Autodesk Inventor part; units mm, degrees
ref_plane "YZ Plane" through (0, 0, 0) normal (1, 0, 0) x (0, 1, 0)
ref_plane "XZ Plane" through (0, 0, 0) normal (0, 1, 0) x (-1, 0, 0)
ref_plane "XY Plane" through (0, 0, 0) normal (0, 0, 1) x (1, 0, 0)
sketch "Block1" plane through (0, 0, 0) normal (0, 0, 1) x (1, 0, 0)
  line L0 (-23.62, 29.22) -> (-7.58, 29.22)
  line L1 (-7.58, 29.22) -> (-7.58, 20.22)
  line L2 (-7.58, 20.22) -> (7.58, 20.22)
  line L3 (7.58, 20.22) -> (7.58, 29.22)
  line L4 (7.58, 29.22) -> (23.62, 29.22)
  line L5 (23.62, 29.22) -> (23.62, 20.22)
  line L6 (23.62, 20.22) -> (39.22, 20.22)
  line L7 (39.22, 20.22) -> (39.22, 13.1133)
  line L8 (39.22, 13.1133) -> (30.22, 13.1133)
  line L9 (30.22, 13.1133) -> (30.22, 5.5533)
  line L10 (30.22, 5.5533) -> (39.22, 5.5533)
  line L11 (39.22, 5.5533) -> (39.22, -5.5533)
  line L12 (39.22, -5.5533) -> (30.22, -5.5533)
  line L13 (30.22, -5.5533) -> (30.22, -13.1133)
  line L14 (30.22, -13.1133) -> (39.22, -13.1133)
  line L15 (39.22, -13.1133) -> (39.22, -20.22)
  line L16 (39.22, -20.22) -> (-39.22, -20.22)
  line L17 (-39.22, -20.22) -> (-39.22, -13.1133)
  line L18 (-39.22, -13.1133) -> (-30.22, -13.1133)
  line L19 (-30.22, -13.1133) -> (-30.22, -5.5533)
  line L20 (-30.22, -5.5533) -> (-39.22, -5.5533)
  line L21 (-39.22, -5.5533) -> (-39.22, 5.5533)
  line L22 (-39.22, 5.5533) -> (-30.22, 5.5533)
  line L23 (-30.22, 5.5533) -> (-30.22, 13.1133)
  line L24 (-30.22, 13.1133) -> (-39.22, 13.1133)
  line L25 (-39.22, 13.1133) -> (-39.22, 20.22)
  line L26 (-39.22, 20.22) -> (-23.62, 20.22)
  line L27 (-23.62, 20.22) -> (-23.62, 29.22)
  line L28 (4.22, 8.55) -> (4.22, 3.11)
  line L29 (4.22, 3.11) -> (-4.22, 3.11)
  line L30 (-4.22, 3.11) -> (-4.22, 8.55)
  line L31 (-4.22, 8.55) -> (4.22, 8.55)
  line L32 (4.22, -3.11) -> (4.22, -8.55)
  line L33 (4.22, -8.55) -> (-4.22, -8.55)
  line L34 (-4.22, -8.55) -> (-4.22, -3.11)
  line L35 (-4.22, -3.11) -> (4.22, -3.11)
  point P0 (0, 5.4933)
sketch "Block2" plane through (0, 0, 0) normal (0, 0, 1) x (1, 0, 0)
  line L0 (-23.5, 29.1) -> (-7.7, 29.1)
  line L1 (-7.7, 29.1) -> (-7.7, 20.1)
  line L2 (-7.7, 20.1) -> (7.7, 20.1)
  line L3 (7.7, 20.1) -> (7.7, 29.1)
  line L4 (7.7, 29.1) -> (23.5, 29.1)
  line L5 (23.5, 29.1) -> (23.5, 20.1)
  line L6 (23.5, 20.1) -> (39.1, 20.1)
  line L7 (39.1, 20.1) -> (39.1, 13.2333)
  line L8 (39.1, 13.2333) -> (30.1, 13.2333)
  line L9 (30.1, 13.2333) -> (30.1, 5.4333)
  line L10 (30.1, 5.4333) -> (39.1, 5.4333)
  line L11 (39.1, 5.4333) -> (39.1, -5.4333)
  line L12 (39.1, -5.4333) -> (30.1, -5.4333)
  line L13 (30.1, -5.4333) -> (30.1, -13.2333)
  line L14 (30.1, -13.2333) -> (39.1, -13.2333)
  line L15 (39.1, -13.2333) -> (39.1, -20.1)
  line L16 (39.1, -20.1) -> (-39.1, -20.1)
  line L17 (-39.1, -20.1) -> (-39.1, -13.2333)
  line L18 (-39.1, -13.2333) -> (-30.1, -13.2333)
  line L19 (-30.1, -13.2333) -> (-30.1, -5.4333)
  line L20 (-30.1, -5.4333) -> (-39.1, -5.4333)
  line L21 (-39.1, -5.4333) -> (-39.1, 5.4333)
  line L22 (-39.1, 5.4333) -> (-30.1, 5.4333)
  line L23 (-30.1, 5.4333) -> (-30.1, 13.2333)
  line L24 (-30.1, 13.2333) -> (-39.1, 13.2333)
  line L25 (-39.1, 13.2333) -> (-39.1, 20.1)
  line L26 (-39.1, 20.1) -> (-23.5, 20.1)
  line L27 (-23.5, 20.1) -> (-23.5, 29.1)
  line L28 (4.1, 8.43) -> (4.1, 3.23)
  line L29 (4.1, 3.23) -> (-4.1, 3.23)
  line L30 (-4.1, 3.23) -> (-4.1, 8.43)
  line L31 (-4.1, 8.43) -> (4.1, 8.43)
  line L32 (4.1, -3.23) -> (4.1, -8.43)
  line L33 (4.1, -8.43) -> (-4.1, -8.43)
  line L34 (-4.1, -8.43) -> (-4.1, -3.23)
  line L35 (-4.1, -3.23) -> (4.1, -3.23)
  point P0 (0, 5.4667)
sketch "Block3" plane through (0, 0, 0) normal (0, 0, 1) x (1, 0, 0)
  line L0 (7.6, 29.2) -> (23.6, 29.2)
  line L1 (23.6, 29.2) -> (23.6, 20.2)
  line L2 (23.6, 20.2) -> (39.2, 20.2)
  line L3 (39.2, 20.2) -> (39.2, 13.1333)
  line L4 (39.2, 13.1333) -> (30.2, 13.1333)
  line L5 (30.2, 13.1333) -> (30.2, 5.5333)
  line L6 (30.2, 5.5333) -> (39.2, 5.5333)
  line L7 (39.2, 5.5333) -> (39.2, -5.5333)
  line L8 (39.2, -5.5333) -> (30.2, -5.5333)
  line L9 (30.2, -5.5333) -> (30.2, -13.1333)
  line L10 (30.2, -13.1333) -> (39.2, -13.1333)
  line L11 (39.2, -13.1333) -> (39.2, -20.2)
  line L12 (39.2, -20.2) -> (-39.2, -20.2)
  line L13 (-39.2, -20.2) -> (-39.2, -13.1333)
  line L14 (-39.2, -13.1333) -> (-30.2, -13.1333)
  line L15 (-30.2, -13.1333) -> (-30.2, -5.5333)
  line L16 (-30.2, -5.5333) -> (-39.2, -5.5333)
  line L17 (-39.2, -5.5333) -> (-39.2, 5.5333)
  line L18 (-39.2, 5.5333) -> (-30.2, 5.5333)
  line L19 (-30.2, 5.5333) -> (-30.2, 13.1333)
  line L20 (-30.2, 13.1333) -> (-39.2, 13.1333)
  line L21 (-39.2, 13.1333) -> (-39.2, 20.2)
  line L22 (-39.2, 20.2) -> (-23.6, 20.2)
  line L23 (-23.6, 20.2) -> (-23.6, 29.2)
  line L24 (-23.6, 29.2) -> (-7.6, 29.2)
  line L25 (-7.6, 29.2) -> (-7.6, 20.2)
  line L26 (-7.6, 20.2) -> (7.6, 20.2)
  line L27 (7.6, 20.2) -> (7.6, 29.2)
  line L28 (4.2, 8.53) -> (4.2, 3.13)
  line L29 (4.2, 3.13) -> (-4.2, 3.13)
  line L30 (-4.2, 3.13) -> (-4.2, 8.53)
  line L31 (-4.2, 8.53) -> (4.2, 8.53)
  line L32 (4.2, -3.13) -> (4.2, -8.53)
  line L33 (4.2, -8.53) -> (-4.2, -8.53)
  line L34 (-4.2, -8.53) -> (-4.2, -3.13)
  line L35 (-4.2, -3.13) -> (4.2, -3.13)
  point P0 (0, 5.4889)
sketch "Block4" plane through (0, 0, 0) normal (0, 0, 1) x (1, 0, 0)
  line L0 (7.7, 29.1) -> (23.5, 29.1)
  line L1 (23.5, 29.1) -> (23.5, 20.1)
  line L2 (23.5, 20.1) -> (39.1, 20.1)
  line L3 (39.1, 20.1) -> (39.1, 13.2333)
  line L4 (39.1, 13.2333) -> (30.1, 13.2333)
  line L5 (30.1, 13.2333) -> (30.1, 5.4333)
  line L6 (30.1, 5.4333) -> (39.1, 5.4333)
  line L7 (39.1, 5.4333) -> (39.1, -5.4333)
  line L8 (39.1, -5.4333) -> (30.1, -5.4333)
  line L9 (30.1, -5.4333) -> (30.1, -13.2333)
  line L10 (30.1, -13.2333) -> (39.1, -13.2333)
  line L11 (39.1, -13.2333) -> (39.1, -20.1)
  line L12 (39.1, -20.1) -> (-39.1, -20.1)
  line L13 (-39.1, -20.1) -> (-39.1, -13.2333)
  line L14 (-39.1, -13.2333) -> (-30.1, -13.2333)
  line L15 (-30.1, -13.2333) -> (-30.1, -5.4333)
  line L16 (-30.1, -5.4333) -> (-39.1, -5.4333)
  line L17 (-39.1, -5.4333) -> (-39.1, 5.4333)
  line L18 (-39.1, 5.4333) -> (-30.1, 5.4333)
  line L19 (-30.1, 5.4333) -> (-30.1, 13.2333)
  line L20 (-30.1, 13.2333) -> (-39.1, 13.2333)
  line L21 (-39.1, 13.2333) -> (-39.1, 20.1)
  line L22 (-39.1, 20.1) -> (-23.5, 20.1)
  line L23 (-23.5, 20.1) -> (-23.5, 29.1)
  line L24 (-23.5, 29.1) -> (-7.7, 29.1)
  line L25 (-7.7, 29.1) -> (-7.7, 20.1)
  line L26 (-7.7, 20.1) -> (7.7, 20.1)
  line L27 (7.7, 20.1) -> (7.7, 29.1)
  line L28 (4.1, 8.43) -> (4.1, 3.23)
  line L29 (4.1, 3.23) -> (-4.1, 3.23)
  line L30 (-4.1, 3.23) -> (-4.1, 8.43)
  line L31 (-4.1, 8.43) -> (4.1, 8.43)
  line L32 (4.1, -3.23) -> (4.1, -8.43)
  line L33 (4.1, -8.43) -> (-4.1, -8.43)
  line L34 (-4.1, -8.43) -> (-4.1, -3.23)
  line L35 (-4.1, -3.23) -> (4.1, -3.23)
  point P0 (0, 5.4667)
sketch "Block5" plane through (0, 0, 0) normal (0, 0, 1) x (1, 0, 0)
  line L0 (-21.38, 25.58) -> (-7.02, 25.58)
  line L1 (-7.02, 25.58) -> (-7.02, 20.08)
  line L2 (-7.02, 20.08) -> (7.02, 20.08)
  line L3 (7.02, 20.08) -> (7.02, 25.58)
  line L4 (7.02, 25.58) -> (21.38, 25.58)
  line L5 (21.38, 25.58) -> (21.38, 20.08)
  line L6 (21.38, 20.08) -> (35.58, 20.08)
  line L7 (35.58, 20.08) -> (35.58, 13.2533)
  line L8 (35.58, 13.2533) -> (30.08, 13.2533)
  line L9 (30.08, 13.2533) -> (30.08, 5.4133)
  line L10 (30.08, 5.4133) -> (35.58, 5.4133)
  line L11 (35.58, 5.4133) -> (35.58, -5.4133)
  line L12 (35.58, -5.4133) -> (30.08, -5.4133)
  line L13 (30.08, -5.4133) -> (30.08, -13.2533)
  line L14 (30.08, -13.2533) -> (35.58, -13.2533)
  line L15 (35.58, -13.2533) -> (35.58, -20.08)
  line L16 (35.58, -20.08) -> (-35.58, -20.08)
  line L17 (-35.58, -20.08) -> (-35.58, -13.2533)
  line L18 (-35.58, -13.2533) -> (-30.08, -13.2533)
  line L19 (-30.08, -13.2533) -> (-30.08, -5.4133)
  line L20 (-30.08, -5.4133) -> (-35.58, -5.4133)
  line L21 (-35.58, -5.4133) -> (-35.58, 5.4133)
  line L22 (-35.58, 5.4133) -> (-30.08, 5.4133)
  line L23 (-30.08, 5.4133) -> (-30.08, 13.2533)
  line L24 (-30.08, 13.2533) -> (-35.58, 13.2533)
  line L25 (-35.58, 13.2533) -> (-35.58, 20.08)
  line L26 (-35.58, 20.08) -> (-21.38, 20.08)
  line L27 (-21.38, 20.08) -> (-21.38, 25.58)
  line L28 (4.08, 8.41) -> (4.08, 3.25)
  line L29 (4.08, 3.25) -> (-4.08, 3.25)
  line L30 (-4.08, 3.25) -> (-4.08, 8.41)
  line L31 (-4.08, 8.41) -> (4.08, 8.41)
  line L32 (4.08, -3.25) -> (4.08, -8.41)
  line L33 (4.08, -8.41) -> (-4.08, -8.41)
  line L34 (-4.08, -8.41) -> (-4.08, -3.25)
  line L35 (-4.08, -3.25) -> (4.08, -3.25)
  point P0 (0, 5.0733)
sketch "Sketch1" plane through (0, 0, 0) normal (0, 0, 1) x (1, 0, 0)
  line L0 (35.5, -20) -> (-35.5, -20)
  line L1 (-35.5, -20) -> (-35.5, 20)
  line L2 (-35.5, 20) -> (35.5, 20)
  line L3 (35.5, 20) -> (35.5, -20)
  line L4 (35.5, -20) -> (-35.5, 20) construction
  line L5 (-35.5, -20) -> (35.5, 20) construction
  point P0 (0, 0)
  point P1 (0, 0)
  dimension "d0" = 71
  dimension "d1" = 40
extrude "Extrusion1" add sketch "Sketch1" against normal blind 5.5
sketch "Sketch3" plane through (0, 0, 0) normal (0, 0, 1) x (1, 0, 0)
  line L0 (-35.5, 20) -> (35.5, 20)
  line L1 (-35.5, -20) -> (-35.5, 20)
  line L2 (-35.5, 13.3333) -> (-30, 13.3333)
  line L3 (-30, 13.3333) -> (-30, 5.3333)
  line L4 (-30, 5.3333) -> (-35.5, 5.3333)
  line L5 (-35.5, 13.3333) -> (-35.5, 5.3333)
  line L6 (-161.1974, 0) -> (72.4829, 0)
  line L7 (0, -29.94) -> (0, 38.94)
  line L8 (35.5, 13.3333) -> (30, 13.3333)
  line L9 (30, 13.3333) -> (30, 5.3333)
  line L10 (30, 5.3333) -> (35.5, 5.3333)
  line L11 (35.5, 13.3333) -> (35.5, 5.3333)
  line L12 (-35.5, -13.3333) -> (-30, -13.3333)
  line L13 (-30, -13.3333) -> (-30, -5.3333)
  line L14 (-30, -5.3333) -> (-35.5, -5.3333)
  line L15 (-35.5, -13.3333) -> (-35.5, -5.3333)
  line L16 (30, -13.3333) -> (30, -5.3333)
  line L17 (35.5, -13.3333) -> (35.5, -5.3333)
  line L18 (30, -5.3333) -> (35.5, -5.3333)
  line L19 (35.5, -13.3333) -> (30, -13.3333)
  point P0 (0, 0)
  dimension "d16" = 5.5
  dimension "d17" = 8
  dimension "d18" = 6.6667
sketch "Sketch4" plane through (0, 0, 0) normal (0, 0, 1) x (1, 0, 0)
  line L0 (4, -8.33) -> (-4, -8.33)
  line L1 (-4, -8.33) -> (-4, -3.33)
  line L2 (-4, -3.33) -> (4, -3.33)
  line L3 (4, -3.33) -> (4, -8.33)
  line L4 (4, -8.33) -> (-4, -3.33) construction
  line L5 (-4, -8.33) -> (4, -3.33) construction
  line L6 (-161.1974, 0) -> (72.4829, 0)
  line L7 (4, 8.33) -> (-4, 8.33)
  line L8 (-4, 8.33) -> (-4, 3.33)
  line L9 (-4, 3.33) -> (4, 3.33)
  line L10 (4, 3.33) -> (4, 8.33)
  line L11 (4, 8.33) -> (-4, 3.33) construction
  line L12 (-4, 8.33) -> (4, 3.33) construction
  point P0 (0, -5.83)
  point P1 (0, 5.83)
  dimension "d25" = 8
  dimension "d26" = 5
  dimension "d27" = 3.33
extrude "Extrusion4" cut sketch "Sketch4" against normal through all
extrude "Extrusion5" cut sketch "Sketch3" against normal through all contours L14 L13 L12 L1 | L2 L3 L4 L1 | L11 L10 L9 L8 | L16 L18 L17 L19
sketch "Sketch5" plane through (0, 0, 0) normal (0, 0, 1) x (1, 0, 0)
  line L0 (-35.5, 20) -> (35.5, 20)
  line L1 (-21.3, 20) -> (-7.1, 20)
  line L2 (-7.1, 20) -> (-7.1, 25.5)
  line L3 (-7.1, 25.5) -> (-21.3, 25.5)
  line L4 (-21.3, 25.5) -> (-21.3, 20)
  line L5 (0, -29.94) -> (0, 38.94)
  line L6 (21.3, 20) -> (7.1, 20)
  line L7 (7.1, 20) -> (7.1, 25.5)
  line L8 (7.1, 25.5) -> (21.3, 25.5)
  line L9 (21.3, 25.5) -> (21.3, 20)
  point P0 (0, 0)
  dimension "d32" = 14.2
  dimension "d33" = 14.2
  dimension "d34" = 5.5
extrude "Extrusion6" add sketch "Sketch5" against normal blind 5.5
equation "\"d2\" = Wt"
equation "\"d16\" = Wt"
equation "\"d17\" = 0.2 * d1"
equation "\"d18\" = 0.166667 * d1"
equation "\"d32\" = 0.2 * d0"
equation "\"d33\" = 0.2 * d0"
equation "\"d34\" = Wt"
equation "\"d35\" = Wt"
equation "\"testKerf1\" = 1"
properties part number "drive_support_side" material "Wood (Birch)"
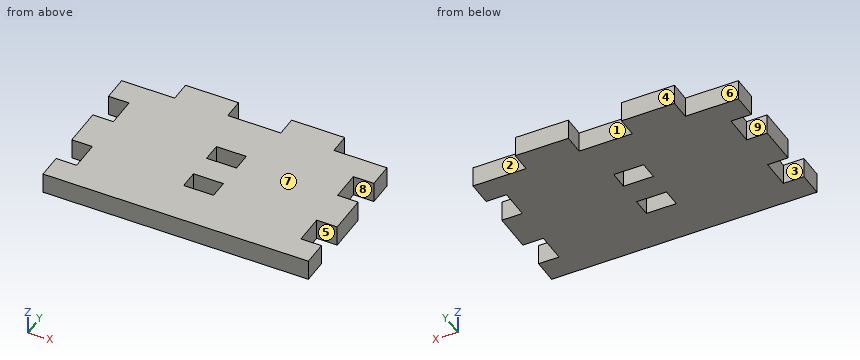
Read the model definition and answer for the solid it produces. Units are mm, in the model's axes. Face numbers are marked on the shaded views. A direction names the side the tool comes from. Round coordinates to 2 decimals unless told otherwise and drop trailing zeros. Loops run counter-clockwise (first coordinate to the right, second up) from the corner with the lowest first, then second, coordinate; pieces in that order, holes last.
Q1. Consider probe 1 along Y at (x, z) = (-3, -4.35); probe 2 along X at (y, z) = (-4, -2.5); probe 3 along X at (y, z) = (-6.5, -2.7). Determine where each line is inside the solid, lowest interval first.
Q2. Section A-A on y = 21 is taken. Write down the section's boundary in (x, z), and give its area (3 significant figures).
Q3. Each of these flat-tipped pins is pushed along its axis until it touches: pin 1 (1.5 mm diameter, centred on y = 6.5, z = -2, fed in from +X); pin 2 (1.6 mm diameter, centred on y = 23, z = -3.5, fed in from -X); pin 3 (1.6 mm diameter, centred on x = 33.5, z = -2, fed in from +Y); pin 4 (3 mm diameter, centred on y = -12, z = -2.5, fed in from +X). Where does it stop, or does it pass through?
Q4. Section D-D on x = -25.5 is taken. Write down the section's boundary in (y, z).
Q5. Section B-B on x = 0 is taken. Write down the section's boundary in (y, z).
Q6. Section C-C on z = -0.8 is taken. Give the number of separate pieces and of enclosed holes in the cut face, and give its area (3 significant figures).
Q7. Determine the mould class of the marked faces 6, 7, 8 and 9 for opening direction Y: released by +Y, released by -Y, zero draft, split by the parting line, or undercut.
Q8. Which of the six approach directions +Z, -Z, +X, -X, +Y, -Y give full straight-line access (tool end or side, diameter ignored) to the marked faces 1, 2, 3, 4 and 5?
Output:
1. probe 1: y = -20 to -8.33, -3.33 to 3.33, 8.33 to 20
1. probe 2: x = -35.5 to -4, 4 to 35.5
1. probe 3: x = -30 to -4, 4 to 30
2. outline: (-21.3, -5.5) - (-7.1, -5.5) - (-7.1, 0) - (-21.3, 0) - close; (7.1, -5.5) - (21.3, -5.5) - (21.3, 0) - (7.1, 0) - close
2. area: 156 mm2
3. pin 1: stops at x = 30
3. pin 2: stops at x = -21.3
3. pin 3: stops at y = 20
3. pin 4: stops at x = 35.5
4. outline: (-20, -5.5) - (20, -5.5) - (20, 0) - (-20, 0) - close
5. outline: (-20, -5.5) - (-8.33, -5.5) - (-8.33, 0) - (-20, 0) - close; (-3.33, -5.5) - (3.33, -5.5) - (3.33, 0) - (-3.33, 0) - close; (8.33, -5.5) - (20, -5.5) - (20, 0) - (8.33, 0) - close
6. separate pieces: 1
6. enclosed holes: 2
6. area: 2,740 mm2
7. face 6: released by +Y
7. face 7: zero draft
7. face 8: undercut
7. face 9: undercut
8. face 1: +Z, -Z, +Y
8. face 2: +Z, -Z, +X, +Y
8. face 3: +Z, -Z, -X
8. face 4: +Z, -Z, +X, -X, +Y
8. face 5: +Z, -Z, +X
